CAD build for the part. Positions are in the model's coordinates, mm. Face numbers are marked on the shaded views. Round coordinates to 2 decimals unless told otherwise and drop trailing zeros. Loops run counter-clockwise (first coordinate to the right, second up) from the corner with the lowest first, then second, coordinate; pieces in that order, holes last. Notation, with made-up numbers: M 66.25,70.5 L 117.25,70.5 A30 cw 117.25,98.5 Z; hole C 43,42.5 d10. An arc over 180 degrees is marked long. Use a Markdown table: item, result. Add a question column.
(1) Wall check: L1, parallel to Y at x = 0, z = 7.5; L2, parallel to Y at x = 0, z = 19.15; L3, parallel to Z at x = 4.5, y = -0.5. Give the ranges that are in metal, low to high.
(2) Band-saw the part on C-C, the plane z = 1.75. Write the cut outline in (x, y).
(3) Two-plate mould, pull along Y, no slides. Class the marked faces 1, 2 and 3: released by +Y, released by -Y, zero draft, split by the parting line, or undercut.
(4) Band-saw the part on A-A, the plane y = 0. Write the cut outline in (x, z), and give its area (3 significant figures).
(5) Flat gauge pins, fed straight in: P1, Ø3, axis at x = -4, z = 11.5, coming from the +Y side; P2, Ø3, axis at x = 6, z = 4.5, coming from the +Y side; P3, Ø4, axis at y = 3.5, z = 12.5, coming from the -X side. Where does each tip first touch, or does it go through?
from build123d import *

# Parameters (mm, degrees)
SKIZZE1_R                       = 8.5
SKIZZE1_R_2                     = 2.9
AUFSATZ_LINEAR_AUSTRAGEN1_DEPTH = 18.65
SKIZZE2_R                       = 8.5
SKIZZE2_R_2                     = 8.15
AUFSATZ_LINEAR_AUSTRAGEN2_DEPTH = 0.6
FASE1_SIZE                      = 0.5


with BuildPart() as part:
    # Skizze1 → Aufsatz-Linear austragen1 (new body)
    with BuildSketch(Plane.XY):
        Circle(SKIZZE1_R)
        Circle(SKIZZE1_R_2, mode=Mode.SUBTRACT)
    extrude(amount=AUFSATZ_LINEAR_AUSTRAGEN1_DEPTH)

    # Skizze2 → Aufsatz-Linear austragen2 (add)
    with BuildSketch(Plane.XY.offset(18.65)):
        Circle(SKIZZE2_R)
        Circle(SKIZZE2_R_2, mode=Mode.SUBTRACT)
    extrude(amount=AUFSATZ_LINEAR_AUSTRAGEN2_DEPTH)

    # Fase1
    fase1_edges = [part.edges().sort_by_distance(p)[0] for p in [
        (-8.5, 0, 0),
        (-2.9, 0, 0),
        (-2.9, 0, 18.65),
    ]]
    chamfer(fase1_edges, length=FASE1_SIZE)


solid = part.part
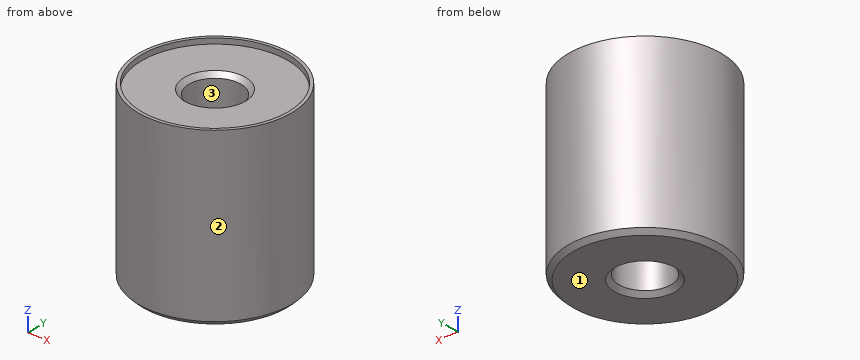
Return value:
| question | item | result |
|---|---|---|
| 1 | L1 | -8.5 to -2.9, 2.9 to 8.5 |
| 1 | L2 | -8.5 to -8.15, 8.15 to 8.5 |
| 1 | L3 | 0 to 18.65 |
| 2 | outline | C 0,0 d17; hole C 0,0 d5.8 |
| 3 | face 1 | zero draft |
| 3 | face 2 | split by the parting line |
| 3 | face 3 | undercut |
| 4 | outline | M -8.5,0.5 L -8,0 L -3.4,0 L -2.9,0.5 L -2.9,18.15 L -3.4,18.65 L -8.15,18.65 L -8.15,19.25 L -8.5,19.25 Z; M 2.9,0.5 L 3.4,0 L 8,0 L 8.5,0.5 L 8.5,19.25 L 8.15,19.25 L 8.15,18.65 L 3.4,18.65 L 2.9,18.15 Z |
| 4 | area | 209 mm^2 |
| 5 | P1 | y = 8.12 |
| 5 | P2 | y = 7.21 |
| 5 | P3 | x = -8.37 |
